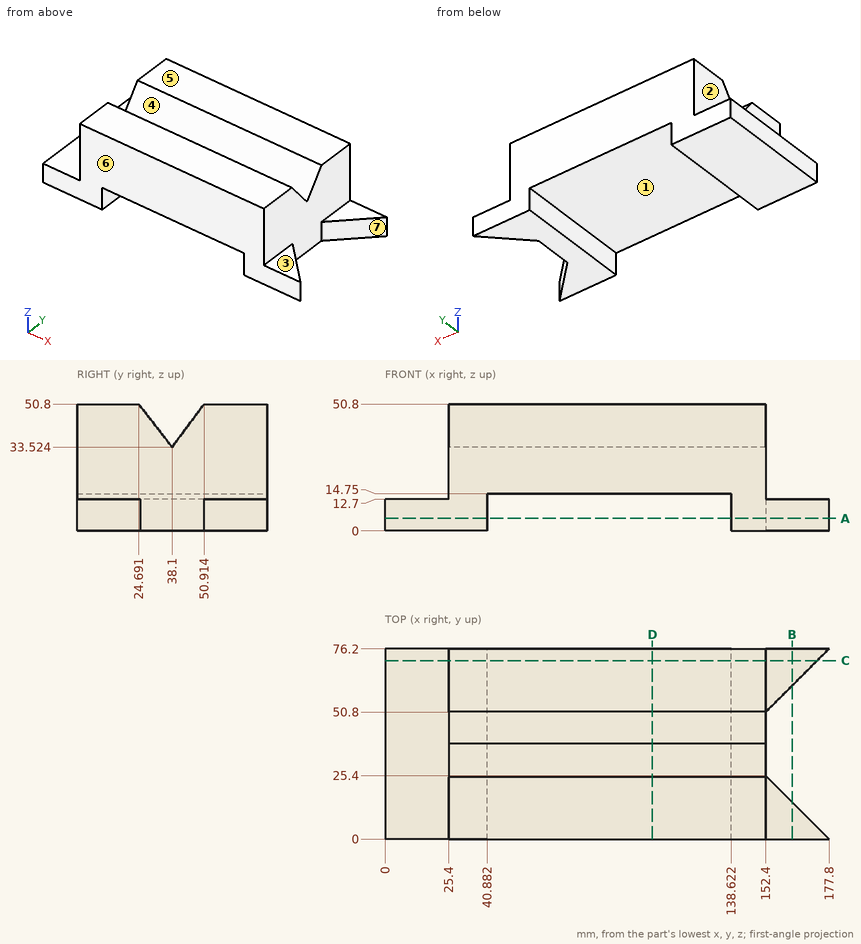
The drawing under review shows one solid part. Ordinate dimensions are in mm from its lowest x, y, z. A direction names the side the tool comes from. Coordinates: 2 decimals unless noted, no trailing zeros. Write each loop counter-clockwise with the first axis right and the second up, starting at its lowest first coordinate (ties: lowest second). Pieces come first, ordered by that corner, then holes. Notation, with made-up numbers: (76.5, 7.5) -> (133.5, 7.5) arc R10 ccw to (133.5, 17.5) -> close; hole circle Ø11 at (30.25, 25). An arc over 180 degrees is marked (long way). One line per item, written item: value. Start each with the question number.
Q1. To check wall thickness, follow probe 1 along X at (y, z) = (43.5, 8); probe 2 along X at (y, z) = (36.5, 14.5); probe 3 along X at (y, z) = (16.5, 21). State the ranges of each line that lie inside material, in increasing order.
Q2. For the marked faces 1, 2 and 3, list the 3-axis set-ups (+Z, -Z, +X, -X, +Y, -Y) from which the entire face can be reached by the end or side of a thin tool; tool diameter is ignored.
Q3. Clearance check with flat-ended pins moving along their axes: P1, Ø20.5, axis at x = 166, y = 62, coming from the +Z side; P2, Ø10, axis at y = 61, z = 38, coming from the +X side; P3, Ø8, axis at x = 147, y = 31, coming from the +Z side (1 decimal). State where each tip first meets the part, or that it passes through.
Q4. The part is to be moulded in two halves that separate along Y. For the marked faces 4, 5, 6 and 7, say which applies: +Y half, -Y half, draft (parallel to the pull), parting line (faces both ways), or undercut.
Q5. Add section D-D, the plane x = 107. Give the boundary of the cut face in (y, z), then the cut area to 3 significant figures.
Q6. Add section C-C, the plane y = 71.5. Give the boundary of the cut face in (x, z).
Q7. Add section A-A, the plane z = 5. Give the boundary of the cut face in (x, y), then the cut area to 3 significant figures.
Q8. Add section B-B, the plane x = 163. Give the boundary of the cut face in (y, z).
Response:
1. probe 1: 0 to 40.88, 138.62 to 152.4
1. probe 2: 25.4 to 40.88, 138.62 to 152.4
1. probe 3: 25.4 to 152.4
2. face 1: -Z, +Y, -Y
2. face 2: +Z, -X, +Y, -Y
2. face 3: +Z, +X, +Y, -Y
3. P1: z = 12.7
3. P2: x = 152.4
3. P3: z = 47.8
4. face 4: undercut
4. face 5: draft
4. face 6: -Y half
4. face 7: undercut
5. outline: (0, 14.75) -> (76.2, 14.75) -> (76.2, 50.8) -> (50.91, 50.8) -> (38.1, 33.52) -> (24.69, 50.8) -> (0, 50.8) -> close
5. area: 2,520 mm²
6. outline: (0, 0) -> (40.88, 0) -> (40.88, 14.75) -> (138.62, 14.75) -> (138.62, 0) -> (173.1, 0) -> (173.1, 12.7) -> (152.4, 12.7) -> (152.4, 50.8) -> (25.4, 50.8) -> (25.4, 12.7) -> (0, 12.7) -> close
7. outline: (0, 0) -> (40.88, 0) -> (40.88, 76.2) -> (0, 76.2) -> close; (138.62, 0) -> (177.8, 0) -> (152.4, 25.4) -> (152.4, 50.8) -> (177.8, 76.2) -> (138.62, 76.2) -> close
7. area: 4,810 mm²
8. outline: (0, 0) -> (14.8, 0) -> (14.8, 12.7) -> (0, 12.7) -> close; (61.4, 0) -> (76.2, 0) -> (76.2, 12.7) -> (61.4, 12.7) -> close
